```python
from build123d import *

# Parameters (mm, degrees)
SKETCH1_R           = 6.35
SKETCH1_R_2         = 2.1336
BOSS_EXTRUDE1_DEPTH = 8.255
CUT_EXTRUDE1_DEPTH  = 19.794283705
SKETCH4_R           = 1.9685
BOSS_EXTRUDE2_DEPTH = 6.985
SKETCH6_W           = 16.51
SKETCH6_H           = 7.62
BOSS_EXTRUDE3_DEPTH = 3.429
FILLET1_R           = 1.27
CHAMFER1_SIZE       = 0.381
SKETCH5_R           = 2.2225
CUT_EXTRUDE2_DEPTH  = 8.255
CHAMFER2_SIZE       = 0.508
FILLET2_R           = 2.54


with BuildPart() as part:
    # Sketch1 → Boss-Extrude1 (new, symmetric)
    with BuildSketch(Plane.XY):
        Circle(SKETCH1_R)
        Circle(SKETCH1_R_2, mode=Mode.SUBTRACT)
    extrude(amount=BOSS_EXTRUDE1_DEPTH, both=True)

    # Sketch3 → Cut-Extrude1 (cut, through all)
    with BuildSketch(Plane.XY.offset(8.255)):
        with BuildLine():
            Line((-4.572, 4.4067353), (-4.572, -4.4067353))
            ThreePointArc((-4.572, -4.4067353), (-6.35, 0), (-4.572, 4.4067353))
        make_face()
        with BuildLine():
            Line((5.08, 3.81), (5.08, -3.81))
            ThreePointArc((5.08, -3.81), (6.35, 0), (5.08, 3.81))
        make_face()
    extrude(amount=-CUT_EXTRUDE1_DEPTH, mode=Mode.SUBTRACT)

    # Sketch4 → Boss-Extrude2 (add)
    with BuildSketch(Plane.ZY.offset(4.572)):
        Circle(SKETCH4_R)
    extrude(amount=BOSS_EXTRUDE2_DEPTH)

    # Sketch6 → Boss-Extrude3 (add)
    with BuildSketch(Plane(origin=(5.08, 0, 0), x_dir=(0, 0, -1), z_dir=(1, 0, 0))):
        Rectangle(SKETCH6_W, SKETCH6_H)
    extrude(amount=BOSS_EXTRUDE3_DEPTH)

    # Fillet1
    fillet1_edges = [part.edges().sort_by_distance(p)[0] for p in [
        (-4.572, 0, -1.9685),
    ]]
    fillet(fillet1_edges, radius=FILLET1_R)

    # Chamfer1
    chamfer1_edges = [part.edges().sort_by_distance(p)[0] for p in [
        (-11.557, 0, -1.9685),
    ]]
    chamfer(chamfer1_edges, length=CHAMFER1_SIZE)

    # Sketch5 → Cut-Extrude2 (cut)
    with BuildSketch(Plane(origin=(8.509, 0, 0), x_dir=(0, 0, -1), z_dir=(1, 0, 0))):
        with Locations((-4.445, 0)):
            Circle(SKETCH5_R)
        with Locations(Location((4.445, 0, 0), (0, 0, 180.000000003))):
            Circle(SKETCH5_R)
    extrude(amount=-CUT_EXTRUDE2_DEPTH, mode=Mode.SUBTRACT)

    # Chamfer2
    chamfer2_edges = [part.edges().sort_by_distance(p)[0] for p in [
        (-2.1336, 0, -8.255),
        (-2.1336, 0, 8.255),
    ]]
    chamfer(chamfer2_edges, length=CHAMFER2_SIZE)

    # Fillet2
    fillet2_edges = [part.edges().sort_by_distance(p)[0] for p in [
        (5.08, 3.81, 0),
        (5.08, -3.81, 0),
    ]]
    fillet(fillet2_edges, radius=FILLET2_R)


solid = part.part
```
The listing builds one solid part. Answer for the finished solid, in the listing's coordinates (mm). A direction names the side the tool comes from. Coordinates: 2 decimals unless noted, no trailing zeros. Write each loop counter-clockwise with the first axis right and the second up, starting at its lowest first coordinate (ties: lowest second). Pieces come first, ordered by that corner, then holes. Notation, with made-up numbers: (69, 49.25) -> (95, 49.25) arc R33 cw to (95, 84.25) -> close; hole circle Ø2 at (2, 22). An arc over 180 degrees is marked (long way). Write each question's results on one line, items separated by ' | '. Start each with the question number.
1) A cutting plane is placed at C-C (z = 7.25). Determine the outline of the cut face in (x, y), then the cut area to 3 significant figures.
2) A tool of negligible diameter and unlimited length cuts with its end or side. For faces 1 (the flat face through (7, -3.81, 0)), 2 (the flat face through (7, 3.81, 0)), 3 (the cylindrical face through (5.357, 0.098, 6.665)), 4 (the cylindrical face through (-8.47, -1.92, -0.43)), from which of +Z, -Z, +X, -X, +Y, -Y can it reach the whole face along a straight path? Write none if from no direction.
3) For a pull along Y with two mould halves and no side action, classify faces 5 (the flat face through (-11.557, 0, 0)), 6 (the cylindrical face through (-0.161, -6.348, 0.116)), 7 (the cylindrical face through (-2.13, 0.09, -0.11)) as +Y half, -Y half, draft (parallel to the pull), parting line (faces both ways), or undercut.
4) A cutting plane is placed at B-B (x = 0). Determine the outline of the cut face in (y, z) (3 decimals), then the cut area to 3 significant figures.
5) Flat-ended cylindrical pins translate along their axes: pin 1 Ø1 at (x, z) = (2, -1) entering from -Y; pin 2 Ø1.8 at (x, z) = (8, -0.5) entering from -Y; pin 3 Ø5 at (x, y) = (0, 0) entering from -Z; pin 4 Ø6 at (y, z) = (0, -4.445) entering from -X. Find the tip coordinate at first contact, or state that the pin passes through.
6) A cutting plane is placed at D-D (z = 3.5). Determine the outline of the cut face in (x, y).
7) A cutting plane is placed at A-A (y = 0). Determine the outline of the cut face in (x, z) (1 decimal), then the cut area to 3 significant figures.
8) Straight lines are drawn through the part: probe 1 along Z at (x, y) = (4.25, 0) (1 decimal); probe 2 along Y at (x, z) = (0, -0.25); probe 3 along Y at (x, z) = (6.25, -1.5). For each, find the intervals that lie inside material, in ascending order.
Values follow:
1) outline: (-4.57, -4.41) arc R6.35 ccw to (4.44, -4.54) arc R2.54 cw to (6.22, -3.81) -> (8.51, -3.81) -> (8.51, 3.81) -> (6.22, 3.81) arc R2.54 cw to (4.44, 4.54) arc R6.35 ccw to (-4.57, 4.41) -> close; hole circle Ø4.27 at (0, 0) | area: 121 mm²
2) face 1: +Z, -Z, +X, -Y | face 2: +Z, -Z, +X, +Y | face 3: +X | face 4: -X
3) face 5: draft | face 6: -Y half | face 7: undercut
4) outline: (-6.35, -8.255) -> (-2.642, -8.255) -> (-2.134, -7.747) -> (-2.134, 7.747) -> (-2.642, 8.255) -> (-6.35, 8.255) -> close; (2.134, -7.747) -> (2.642, -8.255) -> (6.35, -8.255) -> (6.35, 8.255) -> (2.642, 8.255) -> (2.134, 7.747) -> close | area: 139 mm²
5) pin 1: y = -6.17 | pin 2: y = -3.81 | pin 3: z = -8.11 | pin 4: x = -11.56
6) outline: (-4.57, -4.41) arc R6.35 ccw to (4.44, -4.54) arc R2.54 cw to (6.22, -3.81) -> (8.51, -3.81) -> (8.51, -2.01) -> (0.71, -2.01) arc R2.13 cw (long way) to (0.71, 2.01) -> (8.51, 2.01) -> (8.51, 3.81) -> (6.22, 3.81) arc R2.54 cw to (4.44, 4.54) arc R6.35 ccw to (-4.57, 4.41) -> close
7) outline: (-11.6, -1.6) -> (-11.2, -2) -> (-5.8, -2) arc R1.3 cw to (-4.6, -3.2) -> (-4.6, -8.3) -> (-2.6, -8.3) -> (-2.1, -7.7) -> (-2.1, 7.7) -> (-2.6, 8.3) -> (-4.6, 8.3) -> (-4.6, 3.2) arc R1.3 cw to (-5.8, 2) -> (-11.2, 2) -> (-11.6, 1.6) -> close; (2.1, -7.7) -> (2.6, -8.3) -> (8.5, -8.3) -> (8.5, -6.7) -> (2.1, -6.7) -> close; (2.1, -2.2) -> (8.5, -2.2) -> (8.5, 2.2) -> (2.1, 2.2) -> close; (2.1, 6.7) -> (8.5, 6.7) -> (8.5, 8.3) -> (2.6, 8.3) -> (2.1, 7.7) -> close | area: 116 mm²
8) probe 1: -8.3 to -6.7, -2.2 to 2.2, 6.7 to 8.3 | probe 2: -6.35 to -2.13, 2.13 to 6.35 | probe 3: -3.81 to 3.81
